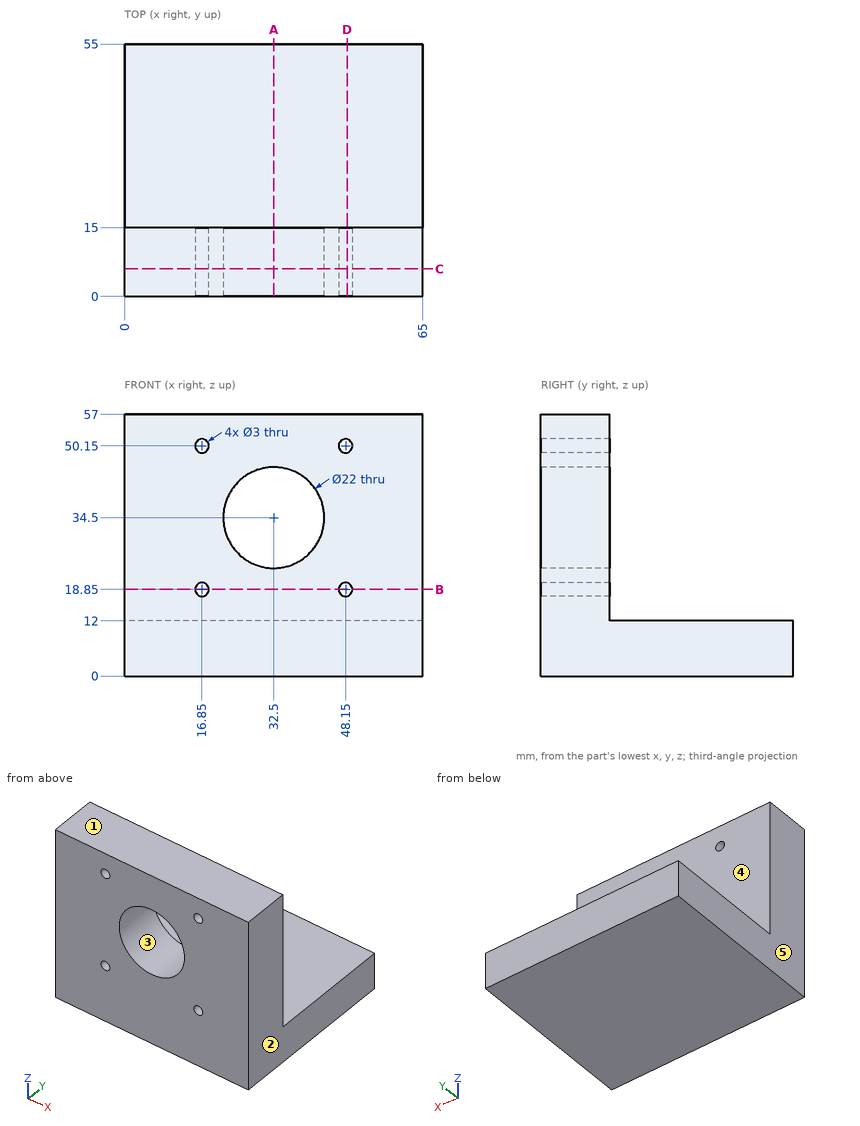
Source: three-view drawing plus pictorial views. Frame: mm from the lowest corner of the part. A direction names the side the tool comes from. Round coordinates to 2 decimals unless told otherwise and drop trailing zeros. Order: outer loops, then holes, each group sorted by start corner. A loop starts at its lowest first (then second) coordinate and runs counter-clockwise, first axis right, second up. Notation, with made-up numbers: M 63,7 L 114,7 A29 cw 114,43 Z; hole C -18,21 d9. An arc over 180 degrees is marked long. One line per item, written item: value.
(1) Cut plane C-C (y = 6). Return the cut outline in (x, z), and give its area (3 significant figures).
Result sheet:
outline: M 0,0 L 65,0 L 65,57 L 0,57 Z; hole C 16.85,18.85 d3; hole C 16.85,50.15 d3; hole C 32.5,34.5 d22; hole C 48.15,18.85 d3; hole C 48.15,50.15 d3
area: 3,300 mm2
(2) Pin query (flat end, axial travel): P1, Ø5, axis at x = 16.85, z = 50.15, coming from the +Y side; P2, Ø13, axis at x = 32.5, z = 34.5, coming from the -Y side; P3, Ø5, axis at x = 35, z = 7, coming from the -Y side; P4, Ø10, axis at x = 58.5, y = 33, coming from the +Z side. Return the tip coordinate at first contact, or that it passes through.
Result sheet:
P1: y = 15
P2: through
P3: y = 0
P4: z = 12
(3) Line query: probe 1 along Z at (x, y) = (48.15, 4); probe 2 along Z at (x, y) = (16, 9); probe 3 along Y at (x, z) = (35, 53.5). Output: solid intervals per line, ascending. Write a range as [from, to].
Result sheet:
probe 1: [0, 17.35], [20.35, 48.65], [51.65, 57]
probe 2: [0, 17.61], [20.09, 48.91], [51.39, 57]
probe 3: [0, 15]
(4) Cut plane D-D (x = 48.5). Return the cut outline in (y, z).
Result sheet:
outline: M 0,0 L 55,0 L 55,12 L 15,12 L 15,17.39 L 0,17.39 Z; M 0,20.31 L 15,20.31 L 15,48.69 L 0,48.69 Z; M 0,51.61 L 15,51.61 L 15,57 L 0,57 Z
(5) Cut plane B-B (z = 18.85). Return the cut outline in (x, y).
Result sheet:
outline: M 0,0 L 15.35,0 L 15.35,15 L 0,15 Z; M 18.35,0 L 46.65,0 L 46.65,15 L 18.35,15 Z; M 49.65,0 L 65,0 L 65,15 L 49.65,15 Z
(6) Reachability of the marked faces 4 and 5 from +Z, -Z, +X, -X, +Y, -Y: full face, straight path, thin tool, end or side. Return the list, or none.
Result sheet:
face 4: +Z, +X, -X, +Y
face 5: +Z, -Z, -X, +Y, -Y
(7) Pull-direction query (X, two-part tool) for the marked faces 1, 2 and 3; classes: pulls with the +X half, pulls with the -X half, needs draft (parallel to the pull), parting line crosses it, or undercut.
Result sheet:
face 1: needs draft
face 2: pulls with the +X half
face 3: undercut
(8) Cut plane A-A (x = 32.5). Return the cut outline in (y, z), and give its area (4 significant figures).
Result sheet:
outline: M 0,0 L 55,0 L 55,12 L 15,12 L 15,23.5 L 0,23.5 Z; M 0,45.5 L 15,45.5 L 15,57 L 0,57 Z
area: 1,005 mm2
